Can you work these out from the model? Positions are in its coordinate system, mm. Give positions to 0.01 mm unless a question says otherwise; leave off trailing zeros. Order: outer loops, then holes, each group sorted by start corner. A loop starts at its lowest first (then second) coordinate and runs counter-clockwise, first axis right, second up.
Item 1: I want a section at A-A, the plane z = 273.5. Write out the boundary of the cut face in (x, y), then the cut area to 3 significant figures.
Item 2: I'm going to push flat-ended pins straight in: pin 1 Ø3 at (x, y) = (-1.5, 4.5) entering from +Z; pin 2 Ø6.5 at (x, z) = (-6.54, 350) entering from +Y; pin 3 Ø8 at (y, z) = (17.5, 834) entering from +X; pin 4 Ø2.5 at (y, z) = (6.5, 654.5) entering from +X. Where does each tip first touch, or does it pass through?
Item 3: If I drill on line 1 along X through (y, z) = (1.2, 350); line 2 along X through (y, z) = (10.5, 401); line 3 along Y through (x, z) = (-0.5, 776.5), over which ranges is the centre line in solid material (lowest first)?
Item 4: I want a section at B-B, the plane y = 23.75. Write out the boundary of the cut face in (x, z), then the cut area to 3 significant figures.
```python
from build123d import *

# Parameters (mm, degrees)
BOSS_EXTRUDE1_DEPTH = 1000
CUT_EXTRUDE1_REACH  = 1002.492
SKETCH2_R           = 2


with BuildPart() as part:
    # Sketch1 → Boss-Extrude1 (new body)
    with BuildSketch(Plane.XY):
        with BuildLine():
            Line((19.707457755, 0), (-10.292542245, 0))
            Line((-10.292542245, 0), (-10.292542245, 4))
            Line((-10.292542245, 4), (-1.292542245, 4))
            Line((-1.292542245, 4), (-1.292542245, 11.8))
            Line((-1.292542245, 11.8), (2.107457755, 17))
            ThreePointArc((2.107457755, 17), (4.707457755, 28.407402334), (7.307457755, 17))
            Line((7.307457755, 17), (10.707457755, 11.8))
            Line((10.707457755, 11.8), (10.707457755, 4))
            Line((10.707457755, 4), (19.707457755, 4))
            Line((19.707457755, 4), (19.707457755, 0))
        make_face()
    extrude(amount=BOSS_EXTRUDE1_DEPTH)

    # Sketch2 → Cut-Extrude1 (cut, up to next)
    with BuildSketch(Plane(origin=(0, 4, 0), x_dir=(1, 0, 0), z_dir=(0, 1, 0)), mode=Mode.PRIVATE) as cut_extrude1_sk1:
        with Locations(Location((-6.542542245, -50, 0), (0, 0, 180))):
            Circle(SKETCH2_R)
    cut_extrude1_tool1 = extrude(cut_extrude1_sk1.sketch, amount=-CUT_EXTRUDE1_REACH, mode=Mode.PRIVATE) & part.part
    # Sketch2 → Cut-Extrude1 (cut, up to next)
    with BuildSketch(Plane(origin=(0, 4, 0), x_dir=(1, 0, 0), z_dir=(0, 1, 0)), mode=Mode.PRIVATE) as cut_extrude1_sk2:
        with Locations(Location((-6.542542245, -150, 0), (0, 0, 180))):
            Circle(SKETCH2_R)
    cut_extrude1_tool2 = extrude(cut_extrude1_sk2.sketch, amount=-CUT_EXTRUDE1_REACH, mode=Mode.PRIVATE) & part.part
    # Sketch2 → Cut-Extrude1 (cut, up to next)
    with BuildSketch(Plane(origin=(0, 4, 0), x_dir=(1, 0, 0), z_dir=(0, 1, 0)), mode=Mode.PRIVATE) as cut_extrude1_sk3:
        with Locations(Location((-6.542542245, -250, 0), (0, 0, 180))):
            Circle(SKETCH2_R)
    cut_extrude1_tool3 = extrude(cut_extrude1_sk3.sketch, amount=-CUT_EXTRUDE1_REACH, mode=Mode.PRIVATE) & part.part
    # Sketch2 → Cut-Extrude1 (cut, up to next)
    with BuildSketch(Plane(origin=(0, 4, 0), x_dir=(1, 0, 0), z_dir=(0, 1, 0)), mode=Mode.PRIVATE) as cut_extrude1_sk4:
        with Locations(Location((-6.542542245, -350, 0), (0, 0, 180))):
            Circle(SKETCH2_R)
    cut_extrude1_tool4 = extrude(cut_extrude1_sk4.sketch, amount=-CUT_EXTRUDE1_REACH, mode=Mode.PRIVATE) & part.part
    # Sketch2 → Cut-Extrude1 (cut, up to next)
    with BuildSketch(Plane(origin=(0, 4, 0), x_dir=(1, 0, 0), z_dir=(0, 1, 0)), mode=Mode.PRIVATE) as cut_extrude1_sk5:
        with Locations(Location((-6.542542245, -450, 0), (0, 0, 180))):
            Circle(SKETCH2_R)
    cut_extrude1_tool5 = extrude(cut_extrude1_sk5.sketch, amount=-CUT_EXTRUDE1_REACH, mode=Mode.PRIVATE) & part.part
    # Sketch2 → Cut-Extrude1 (cut, up to next)
    with BuildSketch(Plane(origin=(0, 4, 0), x_dir=(1, 0, 0), z_dir=(0, 1, 0)), mode=Mode.PRIVATE) as cut_extrude1_sk6:
        with Locations(Location((-6.542542245, -550, 0), (0, 0, 180))):
            Circle(SKETCH2_R)
    cut_extrude1_tool6 = extrude(cut_extrude1_sk6.sketch, amount=-CUT_EXTRUDE1_REACH, mode=Mode.PRIVATE) & part.part
    # Sketch2 → Cut-Extrude1 (cut, up to next)
    with BuildSketch(Plane(origin=(0, 4, 0), x_dir=(1, 0, 0), z_dir=(0, 1, 0)), mode=Mode.PRIVATE) as cut_extrude1_sk7:
        with Locations(Location((-6.542542245, -650, 0), (0, 0, 180))):
            Circle(SKETCH2_R)
    cut_extrude1_tool7 = extrude(cut_extrude1_sk7.sketch, amount=-CUT_EXTRUDE1_REACH, mode=Mode.PRIVATE) & part.part
    # Sketch2 → Cut-Extrude1 (cut, up to next)
    with BuildSketch(Plane(origin=(0, 4, 0), x_dir=(1, 0, 0), z_dir=(0, 1, 0)), mode=Mode.PRIVATE) as cut_extrude1_sk8:
        with Locations(Location((-6.542542245, -750, 0), (0, 0, 180))):
            Circle(SKETCH2_R)
    cut_extrude1_tool8 = extrude(cut_extrude1_sk8.sketch, amount=-CUT_EXTRUDE1_REACH, mode=Mode.PRIVATE) & part.part
    # Sketch2 → Cut-Extrude1 (cut, up to next)
    with BuildSketch(Plane(origin=(0, 4, 0), x_dir=(1, 0, 0), z_dir=(0, 1, 0)), mode=Mode.PRIVATE) as cut_extrude1_sk9:
        with Locations(Location((-6.542542245, -850, 0), (0, 0, 180))):
            Circle(SKETCH2_R)
    cut_extrude1_tool9 = extrude(cut_extrude1_sk9.sketch, amount=-CUT_EXTRUDE1_REACH, mode=Mode.PRIVATE) & part.part
    # Sketch2 → Cut-Extrude1 (cut, up to next)
    with BuildSketch(Plane(origin=(0, 4, 0), x_dir=(1, 0, 0), z_dir=(0, 1, 0)), mode=Mode.PRIVATE) as cut_extrude1_sk10:
        with Locations(Location((-6.542542245, -950, 0), (0, 0, 180))):
            Circle(SKETCH2_R)
    cut_extrude1_tool10 = extrude(cut_extrude1_sk10.sketch, amount=-CUT_EXTRUDE1_REACH, mode=Mode.PRIVATE) & part.part
    # Sketch2 → Cut-Extrude1 (cut, up to next)
    with BuildSketch(Plane(origin=(0, 4, 0), x_dir=(1, 0, 0), z_dir=(0, 1, 0)), mode=Mode.PRIVATE) as cut_extrude1_sk11:
        with Locations(Location((15.957457755, -50, 0), (0, 0, 180))):
            Circle(SKETCH2_R)
    cut_extrude1_tool11 = extrude(cut_extrude1_sk11.sketch, amount=-CUT_EXTRUDE1_REACH, mode=Mode.PRIVATE) & part.part
    # Sketch2 → Cut-Extrude1 (cut, up to next)
    with BuildSketch(Plane(origin=(0, 4, 0), x_dir=(1, 0, 0), z_dir=(0, 1, 0)), mode=Mode.PRIVATE) as cut_extrude1_sk12:
        with Locations(Location((15.957457755, -150, 0), (0, 0, 180))):
            Circle(SKETCH2_R)
    cut_extrude1_tool12 = extrude(cut_extrude1_sk12.sketch, amount=-CUT_EXTRUDE1_REACH, mode=Mode.PRIVATE) & part.part
    # Sketch2 → Cut-Extrude1 (cut, up to next)
    with BuildSketch(Plane(origin=(0, 4, 0), x_dir=(1, 0, 0), z_dir=(0, 1, 0)), mode=Mode.PRIVATE) as cut_extrude1_sk13:
        with Locations(Location((15.957457755, -250, 0), (0, 0, 180))):
            Circle(SKETCH2_R)
    cut_extrude1_tool13 = extrude(cut_extrude1_sk13.sketch, amount=-CUT_EXTRUDE1_REACH, mode=Mode.PRIVATE) & part.part
    # Sketch2 → Cut-Extrude1 (cut, up to next)
    with BuildSketch(Plane(origin=(0, 4, 0), x_dir=(1, 0, 0), z_dir=(0, 1, 0)), mode=Mode.PRIVATE) as cut_extrude1_sk14:
        with Locations(Location((15.957457755, -350, 0), (0, 0, 180))):
            Circle(SKETCH2_R)
    cut_extrude1_tool14 = extrude(cut_extrude1_sk14.sketch, amount=-CUT_EXTRUDE1_REACH, mode=Mode.PRIVATE) & part.part
    # Sketch2 → Cut-Extrude1 (cut, up to next)
    with BuildSketch(Plane(origin=(0, 4, 0), x_dir=(1, 0, 0), z_dir=(0, 1, 0)), mode=Mode.PRIVATE) as cut_extrude1_sk15:
        with Locations(Location((15.957457755, -450, 0), (0, 0, 180))):
            Circle(SKETCH2_R)
    cut_extrude1_tool15 = extrude(cut_extrude1_sk15.sketch, amount=-CUT_EXTRUDE1_REACH, mode=Mode.PRIVATE) & part.part
    # Sketch2 → Cut-Extrude1 (cut, up to next)
    with BuildSketch(Plane(origin=(0, 4, 0), x_dir=(1, 0, 0), z_dir=(0, 1, 0)), mode=Mode.PRIVATE) as cut_extrude1_sk16:
        with Locations(Location((15.957457755, -550, 0), (0, 0, 180))):
            Circle(SKETCH2_R)
    cut_extrude1_tool16 = extrude(cut_extrude1_sk16.sketch, amount=-CUT_EXTRUDE1_REACH, mode=Mode.PRIVATE) & part.part
    # Sketch2 → Cut-Extrude1 (cut, up to next)
    with BuildSketch(Plane(origin=(0, 4, 0), x_dir=(1, 0, 0), z_dir=(0, 1, 0)), mode=Mode.PRIVATE) as cut_extrude1_sk17:
        with Locations(Location((15.957457755, -650, 0), (0, 0, 180))):
            Circle(SKETCH2_R)
    cut_extrude1_tool17 = extrude(cut_extrude1_sk17.sketch, amount=-CUT_EXTRUDE1_REACH, mode=Mode.PRIVATE) & part.part
    # Sketch2 → Cut-Extrude1 (cut, up to next)
    with BuildSketch(Plane(origin=(0, 4, 0), x_dir=(1, 0, 0), z_dir=(0, 1, 0)), mode=Mode.PRIVATE) as cut_extrude1_sk18:
        with Locations(Location((15.957457755, -750, 0), (0, 0, 180))):
            Circle(SKETCH2_R)
    cut_extrude1_tool18 = extrude(cut_extrude1_sk18.sketch, amount=-CUT_EXTRUDE1_REACH, mode=Mode.PRIVATE) & part.part
    # Sketch2 → Cut-Extrude1 (cut, up to next)
    with BuildSketch(Plane(origin=(0, 4, 0), x_dir=(1, 0, 0), z_dir=(0, 1, 0)), mode=Mode.PRIVATE) as cut_extrude1_sk19:
        with Locations(Location((15.957457755, -850, 0), (0, 0, 180))):
            Circle(SKETCH2_R)
    cut_extrude1_tool19 = extrude(cut_extrude1_sk19.sketch, amount=-CUT_EXTRUDE1_REACH, mode=Mode.PRIVATE) & part.part
    # Sketch2 → Cut-Extrude1 (cut, up to next)
    with BuildSketch(Plane(origin=(0, 4, 0), x_dir=(1, 0, 0), z_dir=(0, 1, 0)), mode=Mode.PRIVATE) as cut_extrude1_sk20:
        with Locations(Location((15.957457755, -950, 0), (0, 0, 180))):
            Circle(SKETCH2_R)
    cut_extrude1_tool20 = extrude(cut_extrude1_sk20.sketch, amount=-CUT_EXTRUDE1_REACH, mode=Mode.PRIVATE) & part.part
    add(cut_extrude1_tool1.solids().sort_by_distance((-6.542542, 4, 50))[0], mode=Mode.SUBTRACT)
    add(cut_extrude1_tool2.solids().sort_by_distance((-6.542542, 4, 150))[0], mode=Mode.SUBTRACT)
    add(cut_extrude1_tool3.solids().sort_by_distance((-6.542542, 4, 250))[0], mode=Mode.SUBTRACT)
    add(cut_extrude1_tool4.solids().sort_by_distance((-6.542542, 4, 350))[0], mode=Mode.SUBTRACT)
    add(cut_extrude1_tool5.solids().sort_by_distance((-6.542542, 4, 450))[0], mode=Mode.SUBTRACT)
    add(cut_extrude1_tool6.solids().sort_by_distance((-6.542542, 4, 550))[0], mode=Mode.SUBTRACT)
    add(cut_extrude1_tool7.solids().sort_by_distance((-6.542542, 4, 650))[0], mode=Mode.SUBTRACT)
    add(cut_extrude1_tool8.solids().sort_by_distance((-6.542542, 4, 750))[0], mode=Mode.SUBTRACT)
    add(cut_extrude1_tool9.solids().sort_by_distance((-6.542542, 4, 850))[0], mode=Mode.SUBTRACT)
    add(cut_extrude1_tool10.solids().sort_by_distance((-6.542542, 4, 950))[0], mode=Mode.SUBTRACT)
    add(cut_extrude1_tool11.solids().sort_by_distance((15.957458, 4, 50))[0], mode=Mode.SUBTRACT)
    add(cut_extrude1_tool12.solids().sort_by_distance((15.957458, 4, 150))[0], mode=Mode.SUBTRACT)
    add(cut_extrude1_tool13.solids().sort_by_distance((15.957458, 4, 250))[0], mode=Mode.SUBTRACT)
    add(cut_extrude1_tool14.solids().sort_by_distance((15.957458, 4, 350))[0], mode=Mode.SUBTRACT)
    add(cut_extrude1_tool15.solids().sort_by_distance((15.957458, 4, 450))[0], mode=Mode.SUBTRACT)
    add(cut_extrude1_tool16.solids().sort_by_distance((15.957458, 4, 550))[0], mode=Mode.SUBTRACT)
    add(cut_extrude1_tool17.solids().sort_by_distance((15.957458, 4, 650))[0], mode=Mode.SUBTRACT)
    add(cut_extrude1_tool18.solids().sort_by_distance((15.957458, 4, 750))[0], mode=Mode.SUBTRACT)
    add(cut_extrude1_tool19.solids().sort_by_distance((15.957458, 4, 850))[0], mode=Mode.SUBTRACT)
    add(cut_extrude1_tool20.solids().sort_by_distance((15.957458, 4, 950))[0], mode=Mode.SUBTRACT)


solid = part.part
```
Results list:
1. outline: (-10.29, 0) - (19.71, 0) - (19.71, 4) - (10.71, 4) - (10.71, 11.8) - (7.31, 17) arc R6 ccw (long way) to (2.11, 17) - (-1.29, 11.8) - (-1.29, 4) - (-10.29, 4) - close
1. area: 369 mm2
2. pin 1: stops at z = 1000
2. pin 2: stops at y = 4
2. pin 3: stops at x = 10.64
2. pin 4: stops at x = 10.71
3. line 1: x = -10.29 to -8.54, -4.54 to 13.96, 17.96 to 19.71
3. line 2: x = -1.29 to 10.71
3. line 3: y = 0 to 13.01, 19.43 to 25.39
4. outline: (-1.14, 0) - (10.56, 0) - (10.56, 1000) - (-1.14, 1000) - close
4. area: 11,700 mm2
